For this review, take the finished solid that the model builds, in its own axes (mm). A direction names the side the tool comes from. Give positions to 0.01 mm unless a question says otherwise; leave off trailing zeros. Loops run counter-clockwise (first coordinate to the right, second up) from the corner with the lowest first, then second, coordinate; pieces in that order, holes last. Notation, with made-up numbers: (83, 64.5) - (109, 64.5) arc R16 cw to (109, 94.5) - close; hole circle Ø9 at (-35.75, 84). An arc over 180 degrees is marked (long way). Answer as CSV lines item,"result".
from build123d import *

# Parameters (mm, degrees)
EXTRUDE_1_DEPTH           = 15
SKETCH_2_R                = 35
EXTRUDE_2_DEPTH           = 2
FILLET_1_R                = 2
HOLE_WIZARD_M48_1_D       = 43
CUT_EXTRUDE_1_DEPTH       = 10
FILLET_2_R                = 2
HOLE_START                = 7
HOLE_WIZARD_1_OUTLINE_R   = 5.5
HOLE_WIZARD_1_DEPTH       = 8
HOLE_WIZARD_1_2_OUTLINE_R = 3.3
HOLE_WIZARD_1_2_DEPTH     = 7


# Read off the part's stored shape, not the designer's step: 孔1
with BuildPart() as part:
    # 草图1 → 凸台-拉伸1 (new body)
    with BuildSketch(Plane.XY):
        with BuildLine():
            Line((-37.5, -123), (37.5, -123))
            ThreePointArc((37.5, -123), (42.449747468, -120.949747468), (44.5, -116))
            Line((44.5, -116), (44.5, 116))
            ThreePointArc((44.5, 116), (42.449747468, 120.949747468), (37.5, 123))
            Line((37.5, 123), (-37.5, 123))
            ThreePointArc((-37.5, 123), (-42.449747468, 120.949747468), (-44.5, 116))
            Line((-44.5, 116), (-44.5, -116))
            ThreePointArc((-44.5, -116), (-42.449747468, -120.949747468), (-37.5, -123))
        make_face()
    extrude(amount=EXTRUDE_1_DEPTH)

    # 草图2 → 凸台-拉伸2 (add)
    with BuildSketch(Plane.XY.offset(15)):
        with Locations((0, -71)):
            Circle(SKETCH_2_R)
    extrude(amount=EXTRUDE_2_DEPTH)

    # 圆角1
    fillet_1_edges = [part.edges().sort_by_distance(p)[0] for p in [
        (42.449747468, 120.949747468, 15),
        (0, 123, 15),
        (-42.449747468, 120.949747468, 15),
        (-44.5, 0, 15),
        (-35, -71, 15),
        (-42.449747468, -120.949747468, 15),
        (0, -123, 15),
        (42.449747468, -120.949747468, 15),
        (44.5, 0, 15),
    ]]
    fillet(fillet_1_edges, radius=FILLET_1_R - 0.0001)  # a hair under: the kernel refuses the full size

    # M48 螺纹孔1 (through all)
    with Locations(Plane.XY.offset(17)):
        with Locations((0, -71)):
            Hole(HOLE_WIZARD_M48_1_D / 2)

    # 草图5 → 切除-拉伸1 (cut)
    with BuildSketch(Plane(origin=(0, 0, 0), x_dir=(-1, 0, 0), z_dir=(0, 0, -1))):
        with BuildLine():
            Line((-25.5, -109), (25.5, -109))
            ThreePointArc((25.5, -109), (29.035533906, -107.535533906), (30.5, -104))
            Line((30.5, -104), (30.5, 104))
            ThreePointArc((30.5, 104), (29.035533906, 107.535533906), (25.5, 109))
            Line((25.5, 109), (-25.5, 109))
            ThreePointArc((-25.5, 109), (-29.035533906, 107.535533906), (-30.5, 104))
            Line((-30.5, 104), (-30.5, -104))
            ThreePointArc((-30.5, -104), (-29.035533906, -107.535533906), (-25.5, -109))
        make_face()
    extrude(amount=-CUT_EXTRUDE_1_DEPTH, mode=Mode.SUBTRACT)

    # 圆角2
    fillet_2_edges = [part.edges().sort_by_distance(p)[0] for p in [
        (-29.035533906, -107.535533906, 10),
        (0, -109, 10),
        (29.035533906, -107.535533906, 10),
        (30.5, 0, 10),
        (29.035533906, 107.535533906, 10),
        (0, 109, 10),
        (-29.035533906, 107.535533906, 10),
        (-30.5, 0, 10),
    ]]
    fillet(fillet_2_edges, radius=FILLET_2_R)

    # 孔1 outline → 孔1 (cut)
    with BuildSketch(Plane.XY.offset(HOLE_START)):
        with Locations((36.5, 0)):
            Circle(HOLE_WIZARD_1_OUTLINE_R)
        with Locations((-36.5, 0)):
            Circle(HOLE_WIZARD_1_OUTLINE_R)
        with Locations((36.5, -115)):
            Circle(HOLE_WIZARD_1_OUTLINE_R)
        with Locations((-36.5, 115)):
            Circle(HOLE_WIZARD_1_OUTLINE_R)
        with Locations((-36.5, -115)):
            Circle(HOLE_WIZARD_1_OUTLINE_R)
        with Locations((36.5, 115)):
            Circle(HOLE_WIZARD_1_OUTLINE_R)
    extrude(amount=HOLE_WIZARD_1_DEPTH, mode=Mode.SUBTRACT)

    # Hole Wizard 1 2 outline → Hole Wizard 1 2 (cut)
    with BuildSketch(Plane.XY):
        with Locations((36.5, 0)):
            Circle(HOLE_WIZARD_1_2_OUTLINE_R)
        with Locations((-36.5, 0)):
            Circle(HOLE_WIZARD_1_2_OUTLINE_R)
        with Locations((36.5, -115)):
            Circle(HOLE_WIZARD_1_2_OUTLINE_R)
        with Locations((-36.5, 115)):
            Circle(HOLE_WIZARD_1_2_OUTLINE_R)
        with Locations((-36.5, -115)):
            Circle(HOLE_WIZARD_1_2_OUTLINE_R)
        with Locations((36.5, 115)):
            Circle(HOLE_WIZARD_1_2_OUTLINE_R)
    extrude(amount=HOLE_WIZARD_1_2_DEPTH, mode=Mode.SUBTRACT)


solid = part.part
1) Insertion check: P1, Ø2, axis at x = -23, y = -93, coming from the -Z side; P2, Ø9, axis at x = -37.5, y = 114, coming from the +Z side. Each pin has a flat end and moves straight along its axis. Give the tip position at first contact, or say it passes through.
From the geometry:
P1,"stops at z = 10"
P2,"stops at z = 15"
2) Machinability: for faces 1 (the cylindrical face through (29.07, -107.5, 3.94)), 2 (the cylindrical face through (-42, 0, 11)), 3 (the cylindrical face through (38.02, 112.07, 3.45)), which of the approach directions +Z, -Z, +X, -X, +Y, -Y give a long, thin tool a straight path to every point of the face, cutting with its end or side? Answer none if there is none.
From the geometry:
face 1,"-Z"
face 2,"+Z"
face 3,"+Z, -Z"
3) Draft analysis for pull direction X (two halves, no side actions). For faces 4 (the cylindrical face through (-29, -107.57, 3.94)), 5 (the cylindrical face through (42.5, 120.9, 6.4)), 6 (the flat face through (-1, 29, 15)), state which applies: pulls with the +X half, pulls with the -X half, needs draft (parallel to the pull), parting line crosses it, or undercut.
From the geometry:
face 4,"undercut"
face 5,"pulls with the +X half"
face 6,"needs draft"
4) Consider section B-B on y = -21.5. Write out the cut boundary in (x, z).
From the geometry:
outline,"(-44.5, 0) - (-30.5, 0) - (-30.5, 8) arc R2 cw to (-28.5, 10) - (28.5, 10) arc R2 cw to (30.5, 8) - (30.5, 0) - (44.5, 0) - (44.5, 13) arc R2 ccw to (42.5, 15) - (-42.5, 15) arc R2 ccw to (-44.5, 13) - close"
5) Wall thickness on line 1 (Y direction, x = -36.5, z = 2.5); line 2 (Y direction, x = 36.5, z = 9.5); line 3 (Y direction, x = 6, z = 7): over which ranges is each line inside the solid? List them lowest first. Write a range as from..to.
From the geometry:
line 1,"y = -123..-118.3, -111.7..-3.3, 3.3..111.7, 118.3..123"
line 2,"y = -123..-120.5, -109.5..-5.5, 5.5..109.5, 120.5..123"
line 3,"y = -123..-109, 109..123"
